The model under review builds one solid part; all positions refer to its coordinate system, in mm. A direction names the side the tool comes from. Coordinates: 2 decimals unless noted, no trailing zeros. Order: outer loops, then holes, each group sorted by start corner. A loop starts at its lowest first (then second) coordinate and runs counter-clockwise, first axis right, second up.
```python
from build123d import *

# Parameters (mm, degrees)
SKETCH_1_R               = 1.6
SKETCH_1_R_2             = 1.5
SKETCH_1_W               = 41
SKETCH_1_H               = 21
EXTRUDE_1_DEPTH          = 14
CUT_EXTRUDE_1_DEPTH      = 87.973011371
CUT_EXTRUDE_1_DEPTH_BACK = 87.973011371
SKETCH_2_W               = 4
SKETCH_2_H               = 20
SKETCH_2_H_2             = 48.3
SKETCH_3_W               = 40
SKETCH_3_H               = 4
EXTRUDE_2_DEPTH          = 6
CUT_EXTRUDE_2_DEPTH      = 74.279789476
CUT_EXTRUDE_2_DEPTH_BACK = 74.279789476
SKETCH_4_R               = 1.55


with BuildPart() as part:
    # 草图1 → 凸台-拉伸1 (new body)
    with BuildSketch(Plane.XY):
        with BuildLine():
            Line((55.461772272, 46.736545732), (-48.365006547, 46.736545732))
            ThreePointArc((-48.365006547, 46.736545732), (-48.408359148, 45.857149327), (-48.436816123, 44.977144959))
            ThreePointArc((-48.436816123, 44.977144959), (-48.447916752, 44.35688949), (-48.451617137, 43.736545732))
            ThreePointArc((-48.451617137, 43.736545732), (-39.718232443, 14.892135528), (-16.451617137, -4.263454268))
            Line((-16.451617137, -4.263454268), (-16.451617137, -8.263454268))
            Line((-16.451617137, -8.263454268), (-16.451617137, -24.263454268))
            Line((-16.451617137, -24.263454268), (23.548382863, -24.263454268))
            Line((23.548382863, -24.263454268), (23.548382863, -8.263454268))
            Line((23.548382863, -8.263454268), (23.548382863, -4.263454268))
            ThreePointArc((23.548382863, -4.263454268), (46.814998168, 14.892135528), (55.548382863, 43.736545732))
            ThreePointArc((55.548382863, 43.736545732), (55.526725705, 45.237170718), (55.461772272, 46.736545732))
        make_face()
        with Locations((-11.451617137, 14.736545732)):
            Circle(SKETCH_1_R, mode=Mode.SUBTRACT)
        with Locations((-11.451617137, 24.736545732)):
            Circle(SKETCH_1_R, mode=Mode.SUBTRACT)
        with Locations((-36.451617137, 36.736545732)):
            Circle(SKETCH_1_R_2, mode=Mode.SUBTRACT)
        with Locations((-16.451617137, 36.736545732)):
            Circle(SKETCH_1_R_2, mode=Mode.SUBTRACT)
        with Locations((13.548382863, 19.736545732)):
            Rectangle(SKETCH_1_W, SKETCH_1_H, mode=Mode.SUBTRACT)
        with Locations((38.548382863, 14.736545732)):
            Circle(SKETCH_1_R, mode=Mode.SUBTRACT)
        with Locations((38.548382863, 24.736545732)):
            Circle(SKETCH_1_R, mode=Mode.SUBTRACT)
        with Locations((3.548382863, 36.736545732)):
            Circle(SKETCH_1_R_2, mode=Mode.SUBTRACT)
        with Locations((23.548382863, 36.736545732)):
            Circle(SKETCH_1_R_2, mode=Mode.SUBTRACT)
        with Locations((43.548382863, 36.736545732)):
            Circle(SKETCH_1_R_2, mode=Mode.SUBTRACT)
    extrude(amount=EXTRUDE_1_DEPTH)

    # 草图2 → 切除-拉伸1 (cut, two sides: drawn at the far end of the back side and taken through both)
    with BuildSketch(Plane(origin=(23.548382863, 0, 0), x_dir=(0, 0, -1), z_dir=(1, 0, 0)).offset(-CUT_EXTRUDE_1_DEPTH_BACK)):
        with Locations((-12, -14.263454268)):
            Rectangle(SKETCH_2_W, SKETCH_2_H)
        with Locations((-12, 19.886545732)):
            Rectangle(SKETCH_2_W, SKETCH_2_H_2)
        with Locations((-2, 19.886545732)):
            Rectangle(SKETCH_2_W, SKETCH_2_H_2)
        with Locations((-2, -14.263454268)):
            Rectangle(SKETCH_2_W, SKETCH_2_H)
    extrude(amount=CUT_EXTRUDE_1_DEPTH + CUT_EXTRUDE_1_DEPTH_BACK, mode=Mode.SUBTRACT)

    # 草图3 → 凸台-拉伸2 (add)
    with BuildSketch(Plane(origin=(0, 0, 4), x_dir=(-1, 0, 0), z_dir=(0, 0, -1))):
        with Locations((-3.548382863, -26.263454268)):
            Rectangle(SKETCH_3_W, SKETCH_3_H)
    extrude(amount=-EXTRUDE_2_DEPTH)

    # 草图4 → 切除-拉伸2 (cut, two sides: drawn at the far end of the back side and taken through both)
    with BuildSketch(Plane(origin=(0, 0, 4), x_dir=(-1, 0, 0), z_dir=(0, 0, -1)).offset(-CUT_EXTRUDE_2_DEPTH_BACK)):
        with Locations((-16.548382863, -9.513454268)):
            Circle(SKETCH_4_R)
        with Locations((9.451617137, -9.513454268)):
            Circle(SKETCH_4_R)
    extrude(amount=CUT_EXTRUDE_2_DEPTH + CUT_EXTRUDE_2_DEPTH_BACK, mode=Mode.SUBTRACT)


solid = part.part
```
(1) Machinability: for faces 4 (the face through (3, 44.037, 12)), 5 (the face through (13, 30.237, 7)), 6 (the face through (3, 45, 0)), 7 (the face through (3, 44.037, 2)), which of the approach directions +Z, -Z, +X, -X, +Y, -Y give a long, thin tool a straight path to every point of the face, cutting with its end or side? Answer none if there is none.
A:
face 4: +Z, +X, -X, -Y
face 5: +Z, -Z
face 6: -Z, +X, -X, +Y, -Y
face 7: -Z, +X, -X, -Y
(2) We need section C-C, the plane y = 21. Write out the cut boundary in (x, z), and give its area (3 significant figures).
A:
outline: (-43.22, 4) - (-6.95, 4) - (-6.95, 10) - (-43.22, 10) - close; (34.05, 4) - (50.31, 4) - (50.31, 10) - (34.05, 10) - close
area: 315 mm2
(3) We need section B-B, the plane z = 11.5. Write out the cut boundary in (x, y) (3 decimals), and give its area (3 significant figures).
A:
outline: (-48.451, 44.037) - (55.548, 44.037) arc R52 ccw to (55.462, 46.737) - (-48.365, 46.737) arc R52 ccw to (-48.437, 44.977) arc R52 ccw to start
area: 281 mm2
(4) Wall thickness on probe 1 along X at (y, z) = (-9.5, 5); probe 2 along Y at (x, z) = (11.5, 9); probe 3 along Z at (x, y) = (48, 35): over which ranges is each line inside the solid? List them lowest first.
A:
probe 1: x = -16.45 to -11, -7.9 to 15, 18.1 to 23.55
probe 2: y = -28.26 to 9.24, 30.24 to 46.74
probe 3: z = 4 to 10
(5) We need section A-A, the plane x = 9.5. Write out the cut boundary in (y, z), and give its area (3 significant figures).
A:
outline: (-28.26, 4) - (9.24, 4) - (9.24, 10) - (-28.26, 10) - close; (30.24, 4) - (44.04, 4) - (44.04, 0) - (46.74, 0) - (46.74, 14) - (44.04, 14) - (44.04, 10) - (30.24, 10) - close
area: 346 mm2
(6) For pin 1 Ø3 at (y, z) = (-15.5, 6.5) entering from -X; pin 2 Ø5 at (y, z) = (10.5, 6.5) entering from -X; pin 3 Ø1.8 at (y, z) = (-10.5, 8) entering from +X, all flat-tipped, find the tip position at first contact; note any pin that passes through.
A:
pin 1: stops at x = -16.45
pin 2: stops at x = -38.4
pin 3: stops at x = 23.55
(7) Draft analysis for pull direction X (two halves, no side actions). For faces 1 (the face through (4, 46.737, 7)), 2 (the face through (15.07, -9.05, 7.04)), 3 (the face through (23.548, -16, 7)), state which applies: released by +X, released by -X, zero draft, split by the parting line, or undercut.
A:
face 1: zero draft
face 2: undercut
face 3: released by +X
(8) We need section D-D, the plane x = -41. Write out the cut boundary in (y, z), and give its area (3 significant figures).
A:
outline: (16.91, 4) - (44.04, 4) - (44.04, 0) - (46.74, 0) - (46.74, 14) - (44.04, 14) - (44.04, 10) - (16.91, 10) - close
area: 201 mm2
